Source: three-view drawing plus pictorial views. Frame: mm from the lowest corner of the part. A direction names the side the tool comes from. Give positions to 0.01 mm unless a question says otherwise; leave off trailing zeros. Loops run counter-clockwise (first coordinate to the right, second up) from the corner with the lowest first, then second, coordinate; pieces in that order, holes last.
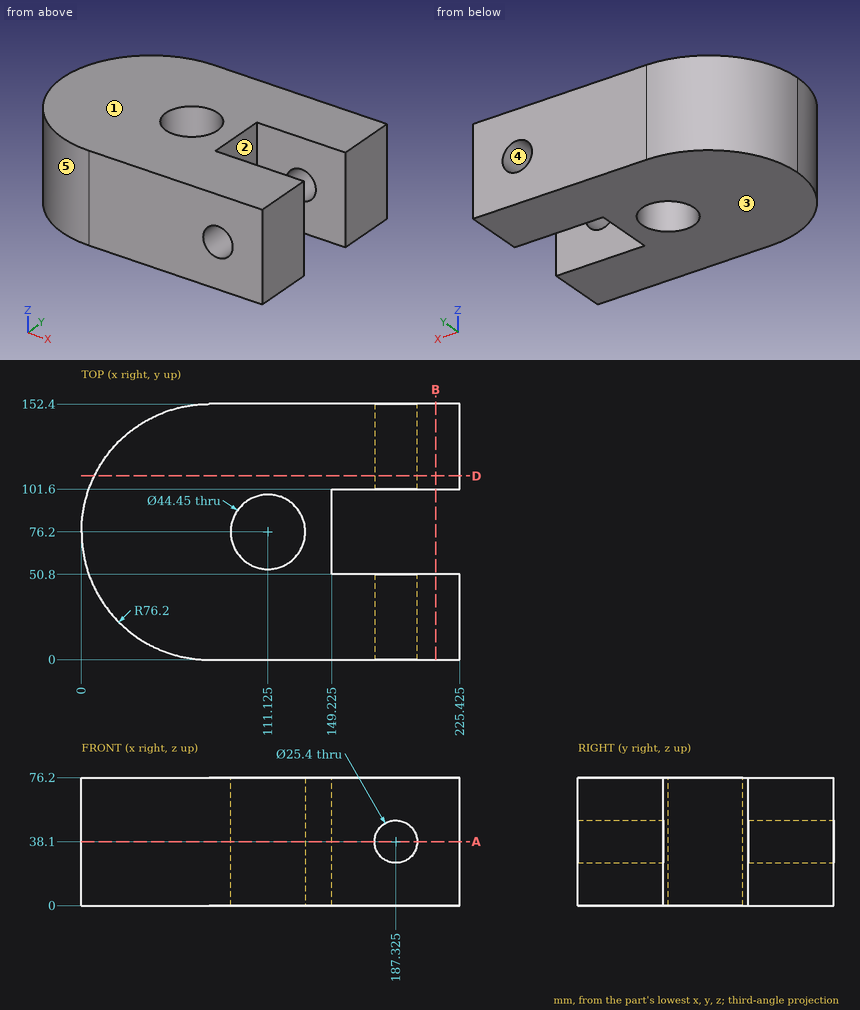
(1) Pin query (flat end, axial travel): pin 1 Ø12 at (x, z) = (30.5, 28.5) entering from +Y; pin 2 Ø3 at (y, z) = (91.5, 42.5) entering from +X (3 decimals); pin 3 Ø23 at (x, z) = (187.325, 38.1) entering from +Y. Return the tip coordinate at first contact, or that it passes through.
Values follow:
pin 1: stops at y = 141.24
pin 2: stops at x = 149.225
pin 3: passes through
(2) Ray query, probe 1 along Y at (x, z) = (156, 44.5); probe 2 along X at (y, z) = (76.5, 22.5) (3 decimals); probe 3 along Y at (x, z) = (103, 9.5). Return the intervals inside material, ascending.
Values follow:
probe 1: y = 0 to 50.8, 101.6 to 152.4
probe 2: x = 0.001 to 88.902, 133.348 to 149.225
probe 3: y = 0 to 55.51, 96.89 to 152.4
(3) Cut plane B-B (x = 211). Return the cut outline in (y, z), and give its area (3 significant figures).
Values follow:
outline: (0, 0) - (50.8, 0) - (50.8, 76.2) - (0, 76.2) - close; (101.6, 0) - (152.4, 0) - (152.4, 76.2) - (101.6, 76.2) - close
area: 7,740 mm2
(4) Cut plane D-D (y = 109.5). Return the cut outline in (x, z) (3 decimals).
Values follow:
outline: (7.661, 0) - (225.425, 0) - (225.425, 76.2) - (7.661, 76.2) - close; hole circle Ø25.4 at (187.325, 38.1)
(5) Cut plane A-A (z = 38.1). Count the separate pieces of the cut face and the enclosed holes in it, and give its area (3 significant figures).
Values follow:
separate pieces: 3
enclosed holes: 1
area: 23,900 mm2
(6) Reachability of the marked faces 1 and 2 from +Z, -Z, +X, -X, +Y, -Y: full face, straight path, thin tool, end or side. Return the list, or none.
Values follow:
face 1: +Z, +X, -X, +Y, -Y
face 2: +Z, -Z, +X
(7) Mould query, pull axis Z, two halves, no side actions, for the marked faces 3, 4 and 5. Classes: +Z half, -Z half, draft (parallel to the pull), parting line (faces both ways), or undercut.
Values follow:
face 3: -Z half
face 4: undercut
face 5: draft
